For this review, use the dimensioned drawing (mm, ordinates from the lowest corner) and the shaded views. A direction names the side the tool comes from. Coordinates: 2 decimals unless noted, no trailing zeros. Order: outer loops, then holes, each group sorted by start corner. A loop starts at its lowest first (then second) coordinate and runs counter-clockwise, first axis right, second up. Notation, with made-up numbers: (86, -10.5) -> (97, -10.5) arc R16 cw to (97, -0.5) -> close; hole circle Ø1 at (18.25, 22). An arc over 180 degrees is marked (long way). Use CSV: the item, a comma, the result in double quotes. Start each with the question number.
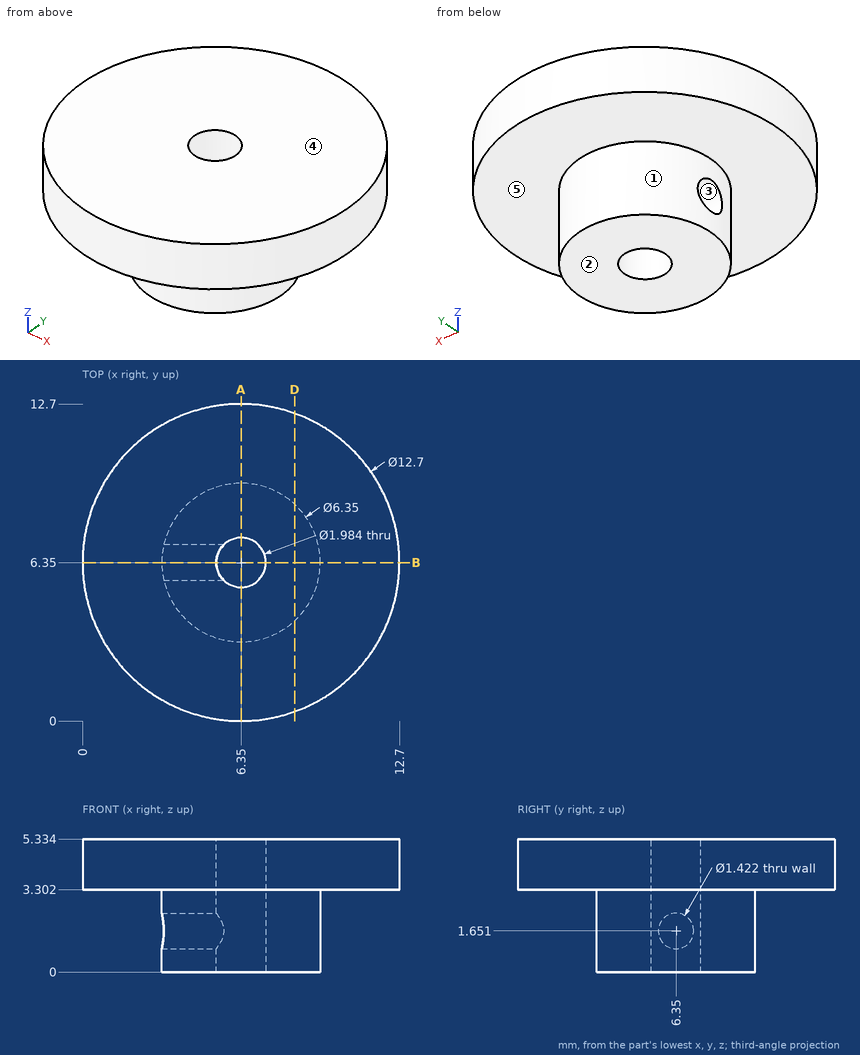
Q1. Add section D-D, the plane x = 8.5. State the section outline as (y, z) points (1 decimal).
Q2. Draft analysis for pull direction Z (two halves, no side actions). For the marked faces 3, 4 and 5, state which applies: +Z half, -Z half, draft (parallel to the pull), parting line (faces both ways), or undercut.
Q3. Add section A-A, the plane x = 6.35. State the section outline as (y, z) points (1 decimal), then the cut area to 3 significant figures.
Q4. Clearance check with flat-ended pins moving along their axes: pin 1 Ø2 at (x, y) = (1.5, 4.5) entering from -Z; pin 2 Ø3 at (x, z) = (3, 3) entering from -Y (1 decimal); pin 3 Ø2.5 at (y, z) = (6.35, 1.651) entering from -X (3 decimals). State where each tip first meets the part, or that it passes through.
Q5. To check wall thickness, follow probe 1 along Y at (x, z) = (6.35, 2.8) (1 decimal); probe 2 along Y at (x, z) = (5.5, 4.4) (1 decimal); probe 3 along Z at (x, y) = (4, 6.25) (1 decimal). State the ranges of each line that lie inside material, in increasing order.
Q6. Add section B-B, the plane y = 6.35. State the section outline as (x, z) points (1 decimal).
Q7. For the marked faces 1 and 2, list the 3-axis set-ups (+Z, -Z, +X, -X, +Y, -Y) from which the entire face can be reached by the end or side of a thin tool; tool diameter is ignored.
Answer block:
1,outline,"(0.4, 3.3) -> (4, 3.3) -> (4, 0) -> (8.7, 0) -> (8.7, 3.3) -> (12.3, 3.3) -> (12.3, 5.3) -> (0.4, 5.3) -> close"
2,face 3,"undercut"
2,face 4,"+Z half"
2,face 5,"-Z half"
3,outline,"(0, 3.3) -> (3.2, 3.3) -> (3.2, 0) -> (5.4, 0) -> (5.4, 5.3) -> (0, 5.3) -> close; (7.3, 0) -> (9.5, 0) -> (9.5, 3.3) -> (12.7, 3.3) -> (12.7, 5.3) -> (7.3, 5.3) -> close"
3,area,"36.2 mm²"
4,pin 1,"stops at z = 3.3"
4,pin 2,"stops at y = 0.3"
4,pin 3,"stops at x = 3.175"
5,probe 1,"y = 3.2 to 5.4, 7.3 to 9.5"
5,probe 2,"y = 0.1 to 5.8, 6.9 to 12.6"
5,probe 3,"z = 0 to 0.9, 2.4 to 5.3"
6,outline,"(0, 3.3) -> (3.2, 3.3) -> (3.2, 2.4) -> (5.4, 2.4) -> (5.4, 5.3) -> (0, 5.3) -> close; (3.2, 0) -> (5.4, 0) -> (5.4, 0.9) -> (3.2, 0.9) -> close; (7.3, 0) -> (9.5, 0) -> (9.5, 3.3) -> (12.7, 3.3) -> (12.7, 5.3) -> (7.3, 5.3) -> close"
7,face 1,"-Z"
7,face 2,"-Z, +X, -X, +Y, -Y"
